Source: three-view drawing plus pictorial views. Frame: mm from the lowest corner of the part. Coordinates: 2 decimals unless noted, no trailing zeros. Order: outer loops, then holes, each group sorted by start corner. A loop starts at its lowest first (then second) coordinate and runs counter-clockwise, first axis right, second up. Notation, with made-up numbers: M -10.75,29.5 L 8.25,29.5 A11 ccw 8.25,33.5 Z; hole C 56,67.5 d6. An arc over 180 degrees is marked long. Use CSV: the item, a comma, the result in double quotes. Start each with the question number.
Q1. Section query A-A, the plane x = 10. Output: boundary loops of the cut face in (y, z), and give its area (3 significant figures).
Q2. First-contact query: P1, Ø1.5, axis at x = 12.5, y = 5, coming from the +Z side. Flat tip, straight axial feed; report the tip coordinate or a pass-through.
Q3. Section query B-B, the plane z = 2.25. Output: boundary loops of the cut face in (x, y), and give its area (3 significant figures).
Q4. Mould query, pull axis X, two halves, no side actions, for the marked faces 1, 2, 3 and 4. Classes: +X half, -X half, draft (parallel to the pull), parting line (faces both ways), or undercut.
Q5. Ray query, probe 1 along Y at (x, z) = (10, 1.2); probe 2 along X at (y, z) = (4.75, 1.7) (1 decimal); probe 3 along X at (y, z) = (10.25, 0.7). Return the intervals inside material, ascending.
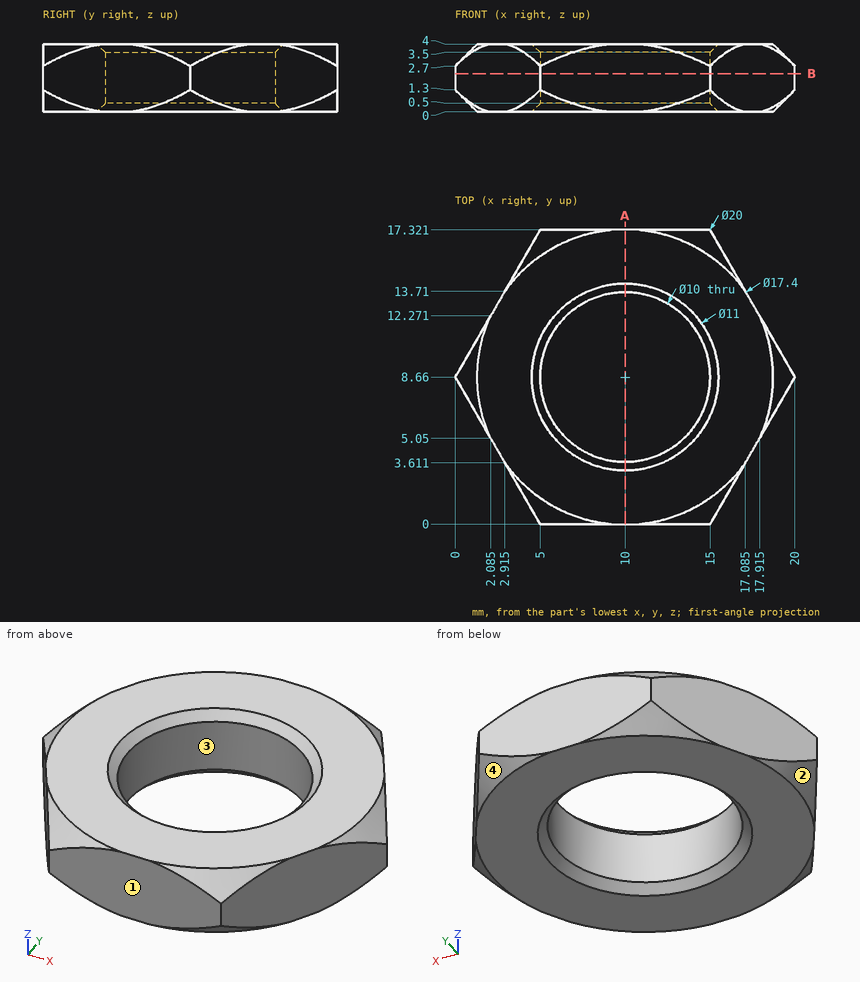
Responses:
1,outline,"M 0,0 L 3.16,0 L 3.66,0.5 L 3.66,3.5 L 3.16,4 L 0,4 Z; M 13.66,0.5 L 14.16,0 L 17.32,0 L 17.32,4 L 14.16,4 L 13.66,3.5 Z"
1,area,"28.8 mm²"
2,P1,"stops at z = 3.68"
3,outline,"M 0,8.66 L 5,0 L 15,0 L 20,8.66 L 15,17.32 L 5,17.32 Z; hole C 10,8.66 d10"
3,area,"181 mm²"
4,face 1,"draft"
4,face 2,"-X half"
4,face 3,"undercut"
4,face 4,"+X half"
5,probe 1,"y = 0 to 3.66, 13.66 to 17.32"
5,probe 2,"x = 2.3 to 6.9, 13.1 to 17.7"
5,probe 3,"x = 0.92 to 5.26, 14.74 to 19.08"
